from build123d import *

# Parameters (mm, degrees)
SKETCH2_W           = 20
SKETCH2_H           = 20
BOSS_EXTRUDE1_DEPTH = 51
SKETCH3_R           = 5
CUT_EXTRUDE1_DEPTH  = 51
SKETCH4_R           = 7.5
BOSS_EXTRUDE2_DEPTH = 40
BOSS_EXTRUDE2_TAPER = 8


with BuildPart() as part:
    # Sketch2 → Boss-Extrude1 (new body)
    with BuildSketch(Plane.XY):
        with Locations((-14.75, 2.75)):
            Rectangle(SKETCH2_W, SKETCH2_H)
    extrude(amount=BOSS_EXTRUDE1_DEPTH)

    # Sketch3 → Cut-Extrude1 (cut)
    with BuildSketch(Plane.XY.offset(51)):
        with Locations((-14.75, 2.75)):
            Circle(SKETCH3_R)
    extrude(amount=-CUT_EXTRUDE1_DEPTH, mode=Mode.SUBTRACT)

    # Sketch4 → Boss-Extrude2 (add)
    with BuildSketch(Plane(origin=(0, 12.75, 0), x_dir=(1, 0, 0), z_dir=(0, 1, 0))):
        with Locations((-14.75, -25.5)):
            Circle(SKETCH4_R)
    extrude(amount=BOSS_EXTRUDE2_DEPTH, taper=BOSS_EXTRUDE2_TAPER)


solid = part.part
Geometry: final body of the model. Coordinates: model frame, mm. Give positions to 0.01 mm unless a question says otherwise; leave off trailing zeros. Loops run counter-clockwise (first coordinate to the right, second up) from the corner with the lowest first, then second, coordinate; pieces in that order, holes last. Notation, with made-up numbers: (2.25, -14) - (13.25, -14) arc R4 ccw to (13.25, -10) - close; hole circle Ø1 at (-22.5, -35). An arc over 180 degrees is marked (long way). One line per question, with ' | ' between items. Start each with the question number.
(1) Section query A-A on y = 2.75. Return loops of the section in (x, z), then the cut area to 3 significant figures.
(2) Section query C-C on z = 37. Return loops of the section in (x, y), then the cut area to 3 significant figures.
(3) Section query B-B on x = -14.75. Return loops of the section in (y, z).
(4) Pull-direction query (X, two-part tool) for faces 1 (the flat face through (-4.75, 3, 25)), 2 (the cylindrical face through (-15.401, 7.707, 25.857)), 3 (the flat face through (-19.33, 5.11, 0)); classes: released by +X, released by -X, zero draft, split by the parting line, or undercut.
(5) Contact query for flat-ended pins moving along their axis: pin 1 (4 mm diameter, centred on x = -18, z = 12, fed in from +Y); pin 2 (1 mm diameter, centred on x = -15.5, y = 34.5, fed in from +Z); pin 3 (10 mm diameter, centred on y = 29, z = 22.5, fed in from -X). Output: stop coordinate, or through.
(6) Ray query, line 1 (X direction, y = 3, z = 30); line 2 (Y direction, x = -22.75, z = 40.5); line 3 (Y direction, x = -14.75, z = 27). Return the intervals inside material, ascending. Write a range as from..to.
(7) Section query D-D on x = -6.5. Return loops of the section in (y, z), then the cut area to 3 significant figures.
The answers:
1) outline: (-24.75, 0) - (-19.75, 0) - (-19.75, 51) - (-24.75, 51) - close; (-9.75, 0) - (-4.75, 0) - (-4.75, 51) - (-9.75, 51) - close | area: 510 mm2
2) outline: (-24.75, -7.25) - (-4.75, -7.25) - (-4.75, 12.75) - (-24.75, 12.75) - close; hole circle Ø10 at (-14.75, 2.75) | area: 321 mm2
3) outline: (-7.25, 0) - (-2.25, 0) - (-2.25, 51) - (-7.25, 51) - close; (7.75, 0) - (12.75, 0) - (12.75, 18) - (52.75, 23.62) - (52.75, 27.38) - (12.75, 33) - (12.75, 51) - (7.75, 51) - close
4) face 1: released by +X | face 2: undercut | face 3: zero draft
5) pin 1: y = 12.75 | pin 2: z = 29.98 | pin 3: x = -20.55
6) line 1: -24.75..-19.74, -9.76..-4.75 | line 2: -7.25..12.75 | line 3: -7.25..-2.25, 7.75..52.75
7) outline: (-7.25, 0) - (12.75, 0) - (12.75, 51) - (-7.25, 51) - close | area: 1,020 mm2
